The drawing under review shows one solid part. Ordinate dimensions are in mm from its lowest x, y, z. A direction names the side the tool comes from. Coordinates: 2 decimals unless noted, no trailing zeros. Write each loop counter-clockwise with the first axis right and the second up, starting at its lowest first coordinate (ties: lowest second). Pieces come first, ordered by that corner, then holes.
1) For the marked faces 3 and 4, list the 3-axis set-ups (+Z, -Z, +X, -X, +Y, -Y) from which the entire face can be reached by the end or side of a thin tool; tool diameter is ignored.
2) We need section D-D on y = 6. Write out the cut boundary in (x, z) (1 decimal).
3) To check wall thickness, follow line 1 along Z through (x, y) = (4.5, 8.4); line 2 along Y through (x, z) = (6.5, 2.5). State the ranges of each line that lie inside material, in increasing order.
4) We need section A-A on y = 2. Write out the cut boundary in (x, z), then the cut area to 3 significant figures.
5) Mouldability with a two-part tool opening along Z and no side actions: class the marked faces 1 and 2 as pulls with the +Z half, pulls with the -Z half, needs draft (parallel to the pull), parting line crosses it, or undercut.
6) Insertion check: P1, Ø1.5, axis at x = 7.5, z = 6, coming from the -Y side; P2, Ø4, axis at y = 5.5, z = 7, coming from the +X side; P3, Ø1, axis at x = 7.5, y = 1, coming from the +Z side; P4, Ø1.6, axis at x = 3.5, y = 5.5, coming from the -Z side. Each pin has a flat end and moves straight along its axis. Give the tip position at first contact, or say it passes through.
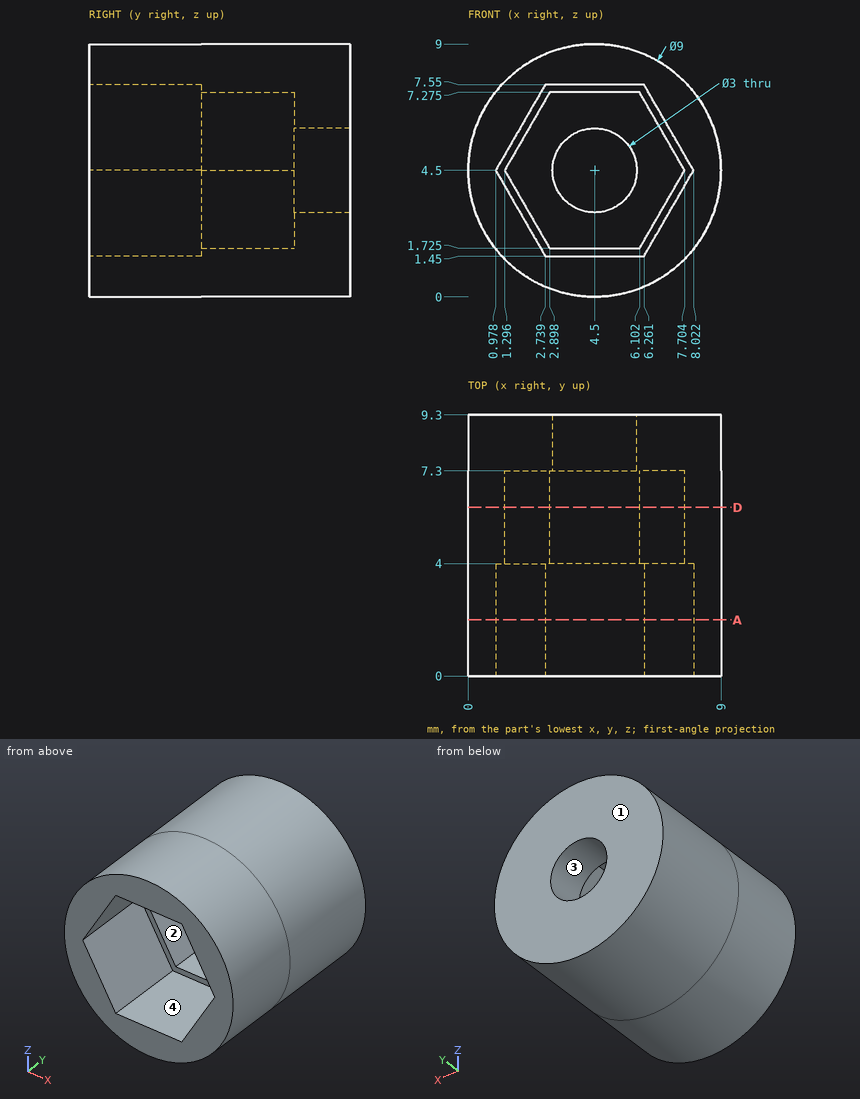
Result:
1. face 3: +Y, -Y
1. face 4: -Y
2. outline: circle Ø9 at (4.5, 4.5); hole (1.3, 4.5) - (2.9, 1.7) - (6.1, 1.7) - (7.7, 4.5) - (6.1, 7.3) - (2.9, 7.3) - close
3. line 1: z = 0 to 3, 6 to 9
3. line 2: y = 7.3 to 9.3
4. outline: circle Ø9 at (4.5, 4.5); hole (0.98, 4.5) - (2.74, 1.45) - (6.26, 1.45) - (8.02, 4.5) - (6.26, 7.55) - (2.74, 7.55) - close
4. area: 31.4 mm2
5. face 1: needs draft
5. face 2: undercut
6. P1: stops at y = 0
6. P2: stops at x = 8.97
6. P3: stops at z = 8.24
6. P4: stops at z = 0
